Check sheet for the modelled part. Datum: model origin and axes. Units: mm. A direction names the side the tool comes from. Round coordinates to 2 decimals unless told otherwise and drop trailing zeros. Write each loop counter-clockwise with the first axis right and the second up, starting at its lowest first coordinate (ties: lowest second). Pieces come first, ordered by that corner, then holes.
Item 1: Set-up check for faces 1 (the flat face through (0, 0, 2.715)), 2 (the flat face through (0, 0, -36.046)), 3 (the flat face through (1.49, -0.01, 3.41)): record each of +Z, -Z, +X, -X, +Y, -Y from which the full face is reachable in a straight line by a thin tool's end or side.
Item 2: Section check C-C, the plane z = 1. Record the cut outline in (x, y).
Item 3: Release check for a two-part mould opening along Y. For faces 4 (the cylindrical face through (1.5, 0.07, -17.31)), 5 (the flat face through (-1, 1, 3.954)), 6 (the flat face through (-1.49, 0.01, 3.41)) record: pulls with the +Y half, pulls with the -Y half, needs draft (parallel to the pull), parting line crosses it, or undercut.
Item 4: Material ranges on line 1 along Z through (x, y) = (0.4, 0.05); line 2 along X through (y, z) = (-0.1, -4), recorded low to high.
Item 5: Section check A-A, the plane x = 0. Record the cut outline in (y, z), plus the area to 3 significant figures.
Item 6: Depth check by flat-ended pin: pin 1 (0.6 mm diameter, centred on y = -1.5, z = 3, fed in from -X); pin 2 (3 mm diameter, centred on y = -0.5, z = -30.5, fed in from -X); pin 3 (0.6 mm diameter, centred on y = 1, z = 3.5, fed in from +X). Enter the tip coordinate at first touch or a pass-through.
Autodesk Inventor part; units mm, degrees
ref_plane "YZ Plane" through (0, 0, 0) normal (1, 0, 0) x (0, 1, 0)
ref_plane "XZ Plane" through (0, 0, 0) normal (0, 1, 0) x (-1, 0, 0)
ref_plane "XY Plane" through (0, 0, 0) normal (0, 0, 1) x (1, 0, 0)
sketch "Sketch1" plane through (0, 0, 0) normal (0, 1, 0) x (-1, 0, 0)
  line L0 (0, 3.9544) -> (2.5, 3.9544)
  line L1 (2.5, 3.9544) -> (1.5, 1.9544)
  line L2 (1.5, 1.9544) -> (1.5, -36.0456)
  line L3 (1.5, -36.0456) -> (0, -36.0456)
  line L4 (0, -36.0456) -> (0, 3.9544)
  point P0 (0, 0)
  dimension "d0" = 2.5
  dimension "d1" = 2
  dimension "d2" = 40
  dimension "d21" = 1.5
revolve "Revolution1" add sketch "Sketch1" angle 360 about axis through (0, 0, -36.0456) along (0, 0, 1)
sketch "Sketch2" plane through (0, 0, 3.9544) normal (0, 0, 1) x (1, 0, 0)
  line L0 (-0.5, 0) -> (0.5, 0)
  line L1 (0.5, 0) -> (0.5, 2)
  line L2 (0.5, 2) -> (-0.5, 2)
  line L3 (-0.5, 2) -> (-0.5, 0)
  point P0 (0, 0)
  dimension "d4" = 1
  dimension "d5" = 2
  dimension "d6" = 0.5
ref_plane "Work Plane2" through (-0.5, 2, 3.9544) normal (-1, 0, 0) x (0, -1, 0)
sketch "Sketch4" plane through (-0.5, 2, 3.9544) normal (-1, 0, 0) x (0, -1, 0)
  line L0 (-0.5, 0) -> (4.5, 0)
  line L1 (-0.4472, 0) -> (0.7164, -1.2393)
  point P0 (2, -3.9544)
  dimension "d15" = 1.7
sweep "Sweep1" cut profiles "Sketch2" path "Sketch4" path curves L1
pattern_circular "Circular Pattern1" count 4 over 360 about axis through (0, 0, 2.9544) along (0, 0, -1) of "Sweep1"
thread "Thread2"
properties part number "Fi3es60mmcsavar" material "Steel, Alloy"
Values found:
1. face 1: none
1. face 2: -Z, +X, -X, +Y, -Y
1. face 3: +Z
2. outline: circle Ø3 at (0, 0)
3. face 4: parting line crosses it
3. face 5: needs draft
3. face 6: undercut
4. line 1: z = -36.05 to 2.72
4. line 2: x = -1.5 to 1.5
5. outline: (-2.5, 3.95) - (-1.5, 1.95) - (-1.5, -36.05) - (1.5, -36.05) - (1.5, 1.95) - (2.5, 3.95) - (2, 3.95) - (1, 2.89) - (1.16, 2.72) - (-1.16, 2.72) - (-1, 2.89) - (-2, 3.95) - close
5. area: 118 mm2
6. pin 1: stops at x = -1.7
6. pin 2: stops at x = -1.5
6. pin 3: stops at x = 2.25
